Part print with two shaded views. Sizes in mm from the minimum x, y, z corner. Give positions to 0.01 mm unless a question says otherwise; leave off trailing zeros. Order: outer loops, then holes, each group sorted by start corner. A loop starts at its lowest first (then second) coordinate and runs counter-clockwise, first axis right, second up.
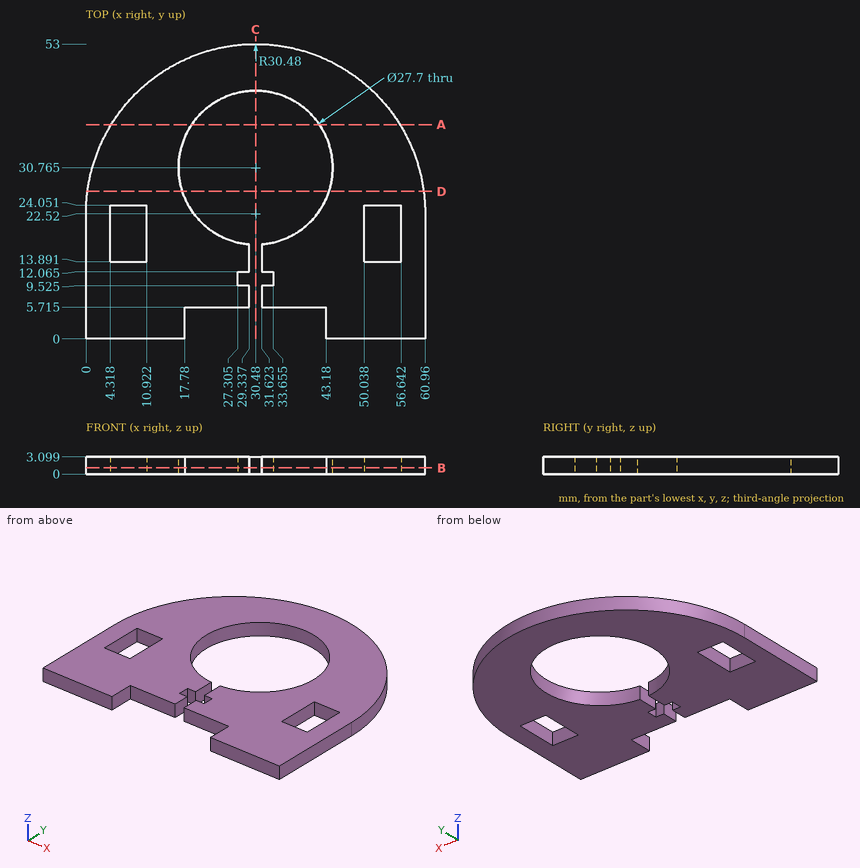
Item 1: Slice it at B-B (z = 1.1). State how many separate pieces and enclosed holes the cut face has, and give its area (3 significant figures).
Item 2: Slice it at A-A (y = 38.5). Give the cut face in (x, z) (1 decimal).
Item 3: Slice it at D-D (y = 26.5). Give the cut face in (x, z).
Item 4: Slice it at C-C (x = 30.48). Give the cut face in (y, z) (1 decimal), and give its area (3 significant figures).
Item 5: Wall check: L1, parallel to X at y = 4, z = 1.15; L2, parallel to X at y = 19, z = 1.05 (1 decimal); L3, parallel to Y at x = 30.48, z = 1.35 (1 decimal). Give the ranges that are in metal, low to high.
Item 6: Drop flat-ended pins along their axis: pin 1 Ø0.9 at (x, z) = (52.5, 1) entering from +Y (1 decimal); pin 2 Ø1.6 at (x, z) = (32.5, 1.5) entering from +Y; pin 3 Ø1.6 at (x, z) = (28.5, 2) entering from -Y (3 decimals). Give the stop position or say it passes through.
A:
1. separate pieces: 1
1. enclosed holes: 2
1. area: 1,910 mm2
2. outline: (4.5, 0) - (19, 0) - (19, 3.1) - (4.5, 3.1) - close; (42, 0) - (56.4, 0) - (56.4, 3.1) - (42, 3.1) - close
3. outline: (0.26, 0) - (17.3, 0) - (17.3, 3.1) - (0.26, 3.1) - close; (43.66, 0) - (60.7, 0) - (60.7, 3.1) - (43.66, 3.1) - close
4. outline: (44.6, 0) - (53, 0) - (53, 3.1) - (44.6, 3.1) - close
4. area: 26.0 mm2
5. L1: x = 0 to 17.78, 43.18 to 60.96
5. L2: x = 0 to 4.3, 10.9 to 23.2, 37.8 to 50, 56.6 to 61
5. L3: y = 44.6 to 53
6. pin 1: stops at y = 44.1
6. pin 2: stops at y = 52.98
6. pin 3: stops at y = 5.715
